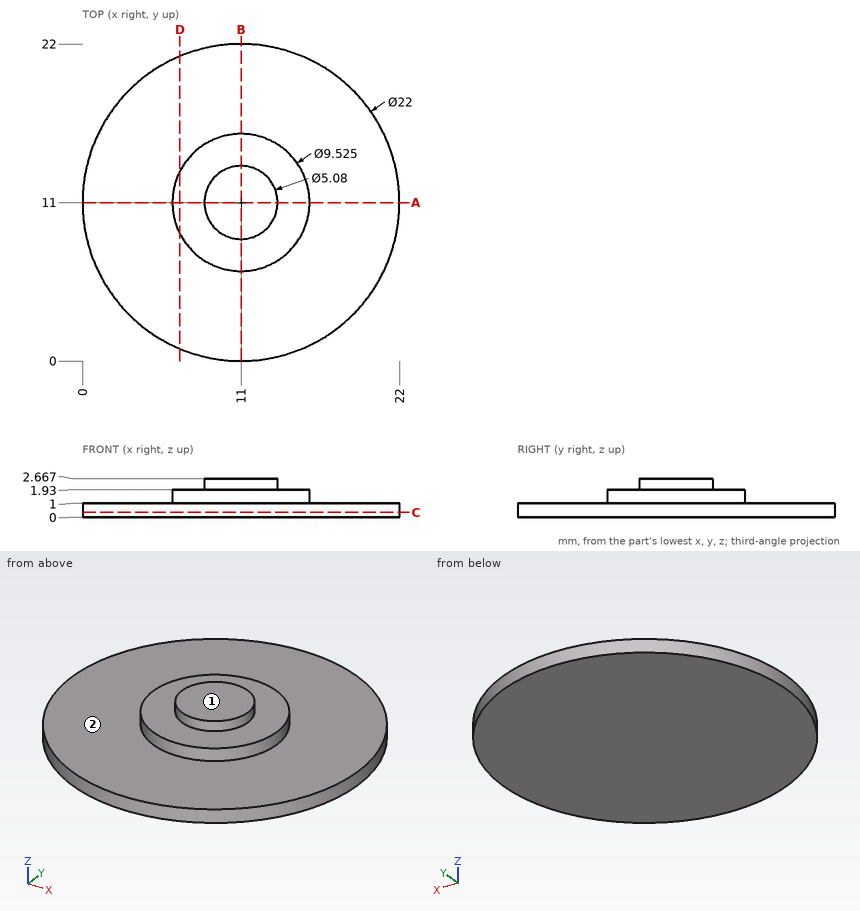
Can you work these out from the drawing? Everything is in mm from the part's minimum corner. A direction names the side the tool comes from. Round coordinates to 2 decimals unless told otherwise and drop trailing zeros. Loops run counter-clockwise (first coordinate to the right, second up) from the corner with the lowest first, then second, coordinate; pieces in that order, holes last. Notation, with made-up numbers: (61, -22.75) - (95, -22.75) arc R18 cw to (95, 2.25) - close; hole circle Ø5 at (-1.75, 3.5). An arc over 180 degrees is marked (long way). Answer in a Markdown table with one row per item. Add a question column.
(1) I need wall thicknesses on line 1 along Z through (x, y) = (3.75, 15); line 2 along Z through (x, y) = (9.25, 8.75); line 3 along X through (y, z) = (8.75, 0.9). Which ranges of each line are inside material? Lowest first, please.
(2) If we section it at C-C (z = 0.35): Please give me the cut outline in (x, y), plus the area to 3 significant figures.
(3) I'm going to push flat-ended pins straight in: pin 1 (8 mm diameter, centred on x = 5.5, y = 19.5, fed in from +Z); pin 2 (5 mm diameter, centred on x = 11, y = 4, fed in from +Z). Where does each tip first touch, or does it pass through?
(4) If we section it at A-A (y = 11): Please give me the cut outline in (x, z), plus the area to 3 significant figures.
(5) For the marked faces 1 and 2, which set-ups out of +Z, -Z, +X, -X, +Y, -Y let a thin tool reach every point of the face, with its end or its side?
(6) If we section it at D-D (x = 6.75): Please give me the cut outline in (y, z).
Model answer:
| question | item | result |
|---|---|---|
| 1 | line 1 | z = 0 to 1 |
| 1 | line 2 | z = 0 to 1.93 |
| 1 | line 3 | x = 0.23 to 21.77 |
| 2 | outline | circle Ø22 at (11, 11) |
| 2 | area | 380 mm² |
| 3 | pin 1 | stops at z = 1 |
| 3 | pin 2 | stops at z = 1.93 |
| 4 | outline | (0, 0) - (22, 0) - (22, 1) - (15.76, 1) - (15.76, 1.93) - (13.54, 1.93) - (13.54, 2.67) - (8.46, 2.67) - (8.46, 1.93) - (6.24, 1.93) - (6.24, 1) - (0, 1) - close |
| 4 | area | 34.6 mm² |
| 5 | face 1 | +Z, +X, -X, +Y, -Y |
| 5 | face 2 | +Z |
| 6 | outline | (0.85, 0) - (21.15, 0) - (21.15, 1) - (13.15, 1) - (13.15, 1.93) - (8.85, 1.93) - (8.85, 1) - (0.85, 1) - close |
